CAD build for the part. Positions are in the model's coordinates, mm. A direction names the side the tool comes from. Round coordinates to 2 decimals unless told otherwise and drop trailing zeros. Order: outer loops, then holes, each group sorted by start corner. A loop starts at its lowest first (then second) coordinate and runs counter-clockwise, first axis right, second up.
```python
from build123d import *

# Parameters (mm, degrees)
F1_DEPTH = 300
F2_T     = -20


with BuildPart() as f1:
    # F0 (on Right) → F1 (new body)
    with BuildSketch(Plane.YZ):
        Polygon((0, 391.622187), (0, 0), (1915.111108, 1606.969024), (1722.274825, 1836.782357), align=None)
    extrude(amount=F1_DEPTH)

    # F2
    f2_openings = [f1.faces().sort_by_distance(p)[0] for p in [
        (150, 0, 195.811093),
        (150, 1818.692966, 1721.875691),
    ]]
    offset(amount=F2_T, openings=f2_openings)


solid = f1.part
```
1. Pin check, flat tips, straight feed: P1, Ø1.5, axis at x = 167, z = 535.5, coming from the +Y side; P2, Ø4, axis at x = 158, y = 685.5, coming from the -Z side; P3, Ø12, axis at x = 51, z = 699, coming from the +Y side. Stop position of each tip, or through.
2. Mould opens along X. For faces 1 (the face through (281, 0, 199)), 2 (the face through (148.18, 937.812, 813.026)), 3 (the face through (0, 882, 991)) say: released by +X, released by -X, zero draft, split by the parting line, or undercut.
3. Cut at C-C, the plane y = 1486.5. Write the cut outline in (x, z).
4. Cut at B-B, the plane z = 1138.5. Write the cut outline in (x, y), and give its area (3 significant figures).
5. Cut at D-D, the plane z = 1714.5. Write the cut outline in (x, y), and give its area (3 significant figures).
6. Drill centre lines: line 1 (X direction, y = 240.5, z = 281); line 2 (Z direction, x = 69, y = 960); line 3 (Y direction, x = 130.5, z = 1078.5). Where is each one in solid material? Low to high.
7. Cut at A-A, the plane x = 119. Write the cut outline in (y, z), and give its area (3 significant figures).
8. Tool access for faces 4 (the face through (280, 876, 928)), 5 (the face through (147.9, 944.15, 792.236)): list every direction of +Z, -Z, +X, -X, +Y, -Y with a clear straight run to the whole face (end or side of a thin tool).
Outcome:
1. P1: stops at y = 639.08
1. P2: stops at z = 573.52
1. P3: stops at y = 840.19
2. face 1: zero draft
2. face 2: undercut
2. face 3: released by -X
3. outline: (0, 1247.32) - (300, 1247.32) - (300, 1638.94) - (0, 1638.94) - close; hole (20, 1273.43) - (280, 1273.43) - (280, 1612.84) - (20, 1612.84) - close
4. outline: (0, 890.09) - (300, 890.09) - (300, 1356.81) - (0, 1356.81) - close; hole (20, 921.21) - (280, 921.21) - (280, 1325.7) - (20, 1325.7) - close
4. area: 34,800 mm2
5. outline: (0, 1576.54) - (300, 1576.54) - (300, 1824.88) - (280, 1824.88) - (280, 1607.66) - (20, 1607.66) - (20, 1824.88) - (0, 1824.88) - close
5. area: 18,000 mm2
6. line 1: x = 0 to 20, 280 to 300
6. line 2: z = 805.54 to 831.64, 1171.05 to 1197.16
6. line 3: y = 818.59 to 849.7, 1254.19 to 1285.31
7. outline: (0, 0) - (1915.11, 1606.97) - (1902.26, 1622.29) - (0, 26.11) - close; (0, 365.51) - (1735.13, 1821.46) - (1722.27, 1836.78) - (0, 391.62) - close
7. area: 95,000 mm2
8. face 4: none
8. face 5: -Z, +X, -X, +Y
